from build123d import *

# Parameters (mm, degrees)
SKETCH_1_W      = 73
SKETCH_1_H      = 8
EXTRUDE_1_DEPTH = 2
SKETCH_1_15_W   = 2.15
SKETCH_1_15_H   = 8
EXTRUDE_2_DEPTH = 20
EXTRUDE_START   = -20
SKETCH_1_16_W   = 6.5
SKETCH_1_16_H   = 8
SKETCH_1_16_R   = 1.5
EXTRUDE_3_DEPTH = 2


with BuildPart() as part:
    # 草图1 → 凸台-拉伸1 (new body)
    with BuildSketch(Plane(origin=(0, 0, 0), x_dir=(1, 0, 0), z_dir=(0, 1, 0))):
        Rectangle(SKETCH_1_W, SKETCH_1_H)
    extrude(amount=EXTRUDE_1_DEPTH)

    # 草图1<15> → 凸台-拉伸2 (add)
    with BuildSketch(Plane(origin=(0, 0, 0), x_dir=(1, 0, 0), z_dir=(0, 1, 0))):
        with Locations((-35.425, 0)):
            Rectangle(SKETCH_1_15_W, SKETCH_1_15_H)
        with Locations((35.425, 0)):
            Rectangle(SKETCH_1_15_W, SKETCH_1_15_H)
    extrude(amount=-EXTRUDE_2_DEPTH)

    # 草图1<16> → 凸台-拉伸3 (add)
    # profile 1 of 2: a face of its own
    with BuildSketch(Plane(origin=(0, 0, 0), x_dir=(1, 0, 0), z_dir=(0, 1, 0)).offset(EXTRUDE_START)):
        with Locations((-39.75, 0)):
            Rectangle(SKETCH_1_16_W, SKETCH_1_16_H)
        with Locations(Location((-39, 0, 0), (0, 0, 270))):
            Circle(SKETCH_1_16_R, mode=Mode.SUBTRACT)
    # profile 2 of 2: a face of its own
    with BuildSketch(Plane(origin=(0, 0, 0), x_dir=(1, 0, 0), z_dir=(0, 1, 0)).offset(EXTRUDE_START)):
        with Locations((39.75, 0)):
            Rectangle(SKETCH_1_16_W, SKETCH_1_16_H)
        with Locations(Location((39, 0, 0), (0, 0, 270))):
            Circle(SKETCH_1_16_R, mode=Mode.SUBTRACT)
    extrude(amount=EXTRUDE_3_DEPTH)


solid = part.part
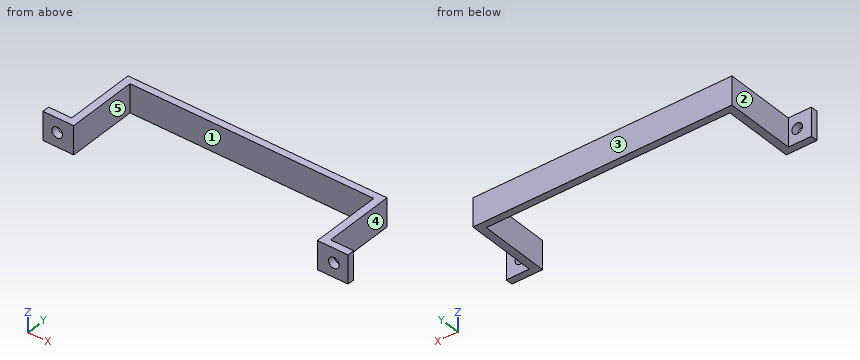
Geometry: final body of the model. Coordinates: model frame, mm. Face numbers are marked on the shaded views. A direction names the side the tool comes from. Coordinates: 2 decimals unless noted, no trailing zeros. Order: outer loops, then holes, each group sorted by start corner. A loop starts at its lowest first (then second) coordinate and runs counter-clockwise, first axis right, second up.
(1) Draft query along X for the marked faces 1, 2 and 3. Return one class per face: pulls with the +X half, pulls with the -X half, needs draft (parallel to the pull), parting line crosses it, or undercut.
(2) First-contact query: pin 1 (2 mm diameter, centred on x = 38.5, z = 1.5, fed in from +Y); pin 2 (2.5 mm diameter, centred on y = -10.5, z = -0.5, fed in from -X); pin 3 (4 mm diameter, centred on y = -7.5, z = -1, fed in from +X). Flat tips, straight axial feed; report the tip coordinate or a pass-through.
(3) Section query B-B (y = -13). Return the cut outline in (x, z).
(4) Section query D-D (x = 4.5). Return the cut outline in (y, z).
(5) Access query for the marked faces 4 and 5. Directions: +Z, -Z, +X, -X, +Y, -Y. A direction counts if a zero-diameter tool reaches every point of the face in a straight line with its end or side. Return the directions, or none.
(6) Section query A-A (x = -39). Return the cut outline in (y, z), plus the area to 3 significant figures.
(7) Material intervals for probe 1 along X at (y, z) = (-19.25, 0); probe 2 along X at (y, z) = (-10.25, -0.25); probe 3 along Y at (x, z) = (13, 3.5), sorted ascending.
(8) Section query C-C (z = 0). Return the cut outline in (x, y), plus the area to 3 significant figures.
Solution:
1. face 1: undercut
1. face 2: pulls with the -X half
1. face 3: needs draft
2. pin 1: stops at y = -18
2. pin 2: stops at x = -36.5
2. pin 3: stops at x = 36.5
3. outline: (-36.5, -4) - (-34.35, -4) - (-34.35, 4) - (-36.5, 4) - close; (34.35, -4) - (36.5, -4) - (36.5, 4) - (34.35, 4) - close
4. outline: (0, -4) - (2, -4) - (2, 4) - (0, 4) - close
5. face 4: +Z, -Z, +X, +Y
5. face 5: +Z, -Z, -Y
6. outline: (-20, -4) - (-18, -4) - (-18, -1.5) - (-20, -1.5) - close; (-20, 1.5) - (-18, 1.5) - (-18, 4) - (-20, 4) - close
6. area: 10.0 mm2
7. probe 1: x = -43 to -40.5, -37.5 to -34.35, 34.35 to 37.5, 40.5 to 43
7. probe 2: x = -36.5 to -34.35, 34.35 to 36.5
7. probe 3: y = 0 to 2
8. outline: (-43, -20) - (-40.5, -20) - (-40.5, -18) - (-43, -18) - close; (-37.5, -20) - (-34.35, -20) - (-34.35, 0) - (34.35, 0) - (34.35, -20) - (37.5, -20) - (37.5, -18) - (36.5, -18) - (36.5, 2) - (-36.5, 2) - (-36.5, -18) - (-37.5, -18) - close; (40.5, -20) - (43, -20) - (43, -18) - (40.5, -18) - close
8. area: 246 mm2
